Autodesk Inventor part; units mm, degrees
ref_plane "YZ Plane" through (0, 0, 0) normal (1, 0, 0) x (0, 1, 0)
ref_plane "XZ Plane" through (0, 0, 0) normal (0, 1, 0) x (-1, 0, 0)
ref_plane "XY Plane" through (0, 0, 0) normal (0, 0, 1) x (1, 0, 0)
ref_plane "Work Plane1" through (170, -244, 0) normal (0, 0, 1) x (1, 0, 0)
sketch "Sketch1" plane through (170, -244, 0) normal (0, 0, 1) x (1, 0, 0)
  line L0 (-170, 244) -> (-180, 244)
  line L1 (-180, 244) -> (-180, 276)
  line L2 (-180, 276) -> (-170, 276)
  line L3 (-170, 276) -> (-170, 244)
  dimension "d0" = 10
  dimension "d1" = 32
extrude "Extrusion1" add sketch "Sketch1" along normal blind 16
sketch "Sketch2" plane through (-10, 0, 0) normal (-1, 0, 0) x (0, 0, 1)
  arc A0 (6, 10) -> (6, 22) centre (6, 16) ccw
  line L0 (0, 32) -> (16, 32)
  line L1 (0, 38.4) -> (0, -6.4)
  line L2 (6, 10) -> (0, 10)
  line L3 (0, 32) -> (0, 0)
  line L4 (6, 22) -> (0, 22)
  line L5 (0, 10) -> (0, 22)
  dimension "d4" = 12
  dimension "d5" = 16
  dimension "d6" = 6
extrude "Extrusion2" cut sketch "Sketch2" against normal blind 16
sketch "Sketch3" plane through (170, -244, 16) normal (0, 0, 1) x (1, 0, 0)
  line L0 (-170, 244) -> (-170, 276)
  line L1 (-170, 276) -> (-180, 276)
  line L2 (-180, 244) -> (-170, 244)
  point P0 (-175, 249)
  point P1 (-175, 271)
  dimension "d9" = 5
  dimension "d10" = 5
  dimension "d11" = 5
  dimension "d12" = 5
hole "Hole1" at (-5, 5, 16) at (-5, 27, 16) direction (0, 0, -1) diameter 6.5 end through all
properties part number "U_OS"
CAD build for the part. Positions are in the model's coordinates, mm. A direction names the side the tool comes from. Give positions to 0.01 mm unless a question says otherwise; leave off trailing zeros. Order: outer loops, then holes, each group sorted by start corner. A loop starts at its lowest first (then second) coordinate and runs counter-clockwise, first axis right, second up. Notation, with made-up numbers: (87, 19.25) - (122, 19.25) arc R7 cw to (122, 32.25) - close; hole circle Ø10 at (-11.75, 51.5). An arc over 180 degrees is marked (long way). Answer in a Markdown table with one row per item.
1. Saw through at B-B, the plane y = 27. Give the cut face in (x, z).
Data:
| item | result |
|---|---|
| outline | (-10, 0) - (-8.25, 0) - (-8.25, 16) - (-10, 16) - close; (-1.75, 0) - (0, 0) - (0, 16) - (-1.75, 16) - close |
2. Probe probe 1 along Y at (x, z) = (-5, 12.25); probe 2 along Y at (x, z) = (-5, 4.5); probe 3 along Y at (x, z) = (-7.75, 8.5). List the from-to ranges inside material, lowest first. Write a range as [from, to].
Data:
| item | result |
|---|---|
| probe 1 | y = [0, 1.75], [8.25, 23.75], [30.25, 32] |
| probe 2 | y = [0, 1.75], [8.25, 10], [22, 23.75], [30.25, 32] |
| probe 3 | y = [0, 3.27], [6.73, 10.55], [21.45, 25.27], [28.73, 32] |
3. Flat gauge pins, fed straight in: pin 1 (6 mm diameter, centred on x = -5, y = 5, fed in from +Z); pin 2 (2 mm diameter, centred on x = -5.5, y = 13.5, fed in from -Z). Where does each tip first touch, or does it go through?
Data:
| item | result |
|---|---|
| pin 1 | passes through |
| pin 2 | stops at z = 10.87 |
4. Saw through at C-C, the plane x = -5. Give the cut face in (y, z).
Data:
| item | result |
|---|---|
| outline | (0, 0) - (1.75, 0) - (1.75, 16) - (0, 16) - close; (8.25, 0) - (10, 0) - (10, 6) arc R6 cw to (22, 6) - (22, 0) - (23.75, 0) - (23.75, 16) - (8.25, 16) - close; (30.25, 0) - (32, 0) - (32, 16) - (30.25, 16) - close |
5. Pull direction Y, two halves, no side cores. Call faces 1 (the flat face through (-5, 10, 3)), 2 (the flat face through (-5, 32, 8)), 3 (the cylindrical face through (-5.98, 23.9, 7.89)), 4 (the flat face through (-5, 0, 8)): pulls with the +Y half, pulls with the -Y half, needs draft (parallel to the pull), parting line crosses it, or undercut.
Data:
| item | result |
|---|---|
| face 1 | undercut |
| face 2 | pulls with the +Y half |
| face 3 | undercut |
| face 4 | pulls with the -Y half |
6. Tool access for faces 5 (the flat face through (-10, 19.3, 11.4)), 6 (the flat face through (-5, 22, 3)): list every direction of +Z, -Z, +X, -X, +Y, -Y with a clear straight run to the whole face (end or side of a thin tool).
Data:
| item | result |
|---|---|
| face 5 | +Z, -Z, -X, +Y, -Y |
| face 6 | -Z, +X, -X |
7. Saw through at D-D, the plane z = 10.75. Give the cut face in (x, y).
Data:
| item | result |
|---|---|
| outline | (-10, 0) - (0, 0) - (0, 12.33) - (-10, 12.33) - close; (-10, 19.67) - (0, 19.67) - (0, 32) - (-10, 32) - close; hole circle Ø6.5 at (-5, 5); hole circle Ø6.5 at (-5, 27) |
8. Saw through at A-A, the plane z = 3. Give the cut face in (x, y).
Data:
| item | result |
|---|---|
| outline | (-10, 0) - (0, 0) - (0, 10) - (-10, 10) - close; (-10, 22) - (0, 22) - (0, 32) - (-10, 32) - close; hole circle Ø6.5 at (-5, 5); hole circle Ø6.5 at (-5, 27) |
